```python
from build123d import *

# Parameters (mm, degrees)
SKETCH_1_R        = 8
SKETCH_1_R_2      = 4
EXTRUDE_1_DEPTH   = 10
EXTRUDE_1_2_DEPTH = 10
EXTRUDE_START     = -1
EXTRUDE_2_DEPTH   = 8
EXTRUDE_START_2   = 1
EXTRUDE_3_DEPTH   = 8
SKETCH_5_R        = 8
SKETCH_5_R_2      = 4
EXTRUDE_4_DEPTH   = 10


with BuildPart() as part:
    # Sketch 1 → Extrude 1 (new body)
    with BuildSketch(Plane.XY):
        Circle(SKETCH_1_R)
        Circle(SKETCH_1_R_2, mode=Mode.SUBTRACT)
    extrude(amount=-EXTRUDE_1_DEPTH)



with BuildPart() as body_2:
    # Sketch 1 → Extrude 1 2 (new body)
    with BuildSketch(Plane.XY):
        with Locations((-53.605968084, 26.951812291)):
            Circle(SKETCH_1_R)
        with Locations((-53.605968084, 26.951812291)):
            Circle(SKETCH_1_R_2, mode=Mode.SUBTRACT)
    extrude(amount=-EXTRUDE_1_2_DEPTH)


with BuildPart() as part_1:
    add(part.part)

    add(body_2.part)  # Extrude 2 merges body 2
    # Sketch 3 → Extrude 2 (add)
    with BuildSketch(Plane.XY.offset(EXTRUDE_START)):
        with BuildLine():
            Line((-51.573547302, 19.214289059), (-7.42278324, -2.983670385))
            ThreePointArc((-7.42278324, -2.983670385), (-7.147462411, 3.593574972), (-2.032420782, 7.737523232))
            Line((-2.032420782, 7.737523232), (-46.183184844, 29.935482676))
            ThreePointArc((-46.183184844, 29.935482676), (-46.458505673, 23.358237319), (-51.573547302, 19.214289059))
        make_face()
    extrude(amount=-EXTRUDE_2_DEPTH)



with BuildPart() as body_2_2:
    # Sketch 4 → Extrude 3 (new body)
    with BuildSketch(Plane.XY.offset(EXTRUDE_START_2)):
        with BuildLine():
            Line((6.92820323, 4), (26.92820323, -30.641016151))
            ThreePointArc((26.92820323, -30.641016151), (33.036798625, -45.545943872), (34.959960983, -61.538856509))
            ThreePointArc((34.959960983, -61.538856509), (41.911210079, -98.657642521), (62.774179905, -130.135581289))
            ThreePointArc((62.774179905, -130.135581289), (62.827441336, -138.566924041), (54.397444356, -138.726699833))
            ThreePointArc((54.397444356, -138.726699833), (26.885397662, -101.001387411), (14.477282647, -55.988604867))
            ThreePointArc((14.477282647, -55.988604867), (11.073298234, -38.952300047), (4.07179677, -23.052558883))
            Line((4.07179677, -23.052558883), (-6.92820323, -4))
            ThreePointArc((-6.92820323, -4), (4, -6.92820323), (6.92820323, 4))
        make_face()
    extrude(amount=EXTRUDE_3_DEPTH)


with BuildPart() as part_2:
    add(part_1.part)

    add(body_2_2.part)  # Extrude 4 merges body 2 2
    # Sketch 5 → Extrude 4 (add)
    with BuildSketch(Plane.XY):
        Circle(SKETCH_5_R)
        Circle(SKETCH_5_R_2, mode=Mode.SUBTRACT)
    extrude(amount=EXTRUDE_4_DEPTH)


solid = part_2.part
```
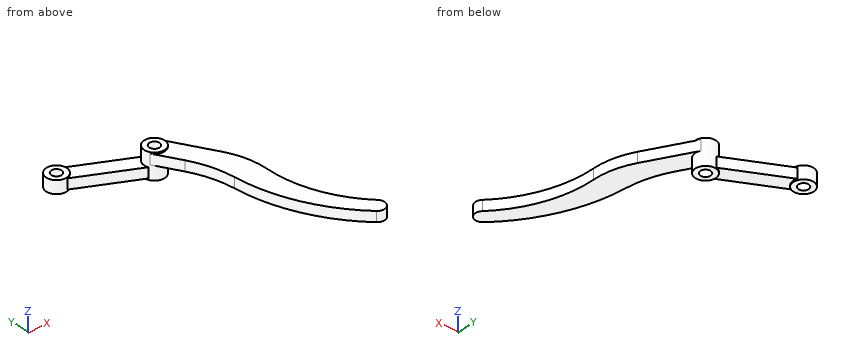
Check sheet for the modelled part. Datum: model origin and axes. Units: mm. Coordinates: 2 decimals unless noted, no trailing zeros. Order: outer loops, then holes, each group sorted by start corner. A loop starts at its lowest first (then second) coordinate and runs counter-clockwise, first axis right, second up. Notation, with made-up numbers: M 6,24 L 42,24 A23 cw 42,58 Z; hole C 28.5,15 d2. An arc over 180 degrees is marked long. One line per question, with ' | ' between items. Start each with the question number.
Item 1: Material ranges on line 1 (Y direction, x = 0, z = -3.5); line 2 (Y direction, x = 0, z = 5.5); line 3 (X direction, y = 2.5, z = 3), recorded low to high.
Item 2: Sectioned sample at A-A on x = 0. Record the cut outline in (y, z).
Item 3: Sectioned sample at C-C on z = 7. Record the cut outline in (x, y), and give its area (3 significant figures).
Item 4: Gauge pin test, flat ends, axial feed: P1, Ø8, axis at x = -52, y = 29.5, coming from the +Z side; P2, Ø5, axis at x = 0, y = 0, coming from the -Z side; P3, Ø16.5, axis at x = -21, y = 6, coming from the -Z side; P4, Ø2, axis at x = 15, z = 5.5, coming from the +Y side. Record the tip position at first contact, or that the pin passes through.
Item 5: Sectioned sample at D-D on z = -4.75. Record the cut outline in (x, y).
Item 6: Sectioned sample at B-B on y = 0. Record the cut outline in (x, z), and give its area (3 significant figures).
Answer below:
1) line 1: y = -8 to -4, 4 to 8 | line 2: y = -16 to -4, 4 to 8 | line 3: x = -7.6 to -3.12, 3.12 to 7.79
2) outline: M -16,1 L -8,1 L -8,-10 L -4,-10 L -4,10 L -8,10 L -8,9 L -16,9 Z; M 4,-10 L 8,-10 L 8,10 L 4,10 Z
3) outline: M -6.93,-4 L 4.07,-23.05 A80 cw 14.48,-55.99 A130 ccw 54.4,-138.73 A6 ccw 62.77,-130.14 A95 cw 34.96,-61.54 A60 ccw 26.93,-30.64 L 6.93,4 A8 ccw Z; hole C 0,0 d8 | area: 2,520 mm^2
4) P1: stops at z = 0 | P2: passes through | P3: stops at z = -9 | P4: stops at y = -8.25
5) outline: M -51.57,19.21 L -7.42,-2.98 A8 ccw long -2.03,7.74 L -46.18,29.94 A8 ccw long Z; hole C -53.61,26.95 d8; hole C 0,0 d8
6) outline: M -13.36,-9 L -8,-9 L -8,-10 L -4,-10 L -4,10 L -8,10 L -8,-1 L -13.36,-1 Z; M 4,-10 L 8,-10 L 8,1 L 9.24,1 L 9.24,9 L 8,9 L 8,10 L 4,10 Z | area: 213 mm^2
